For this review, use the dimensioned drawing (mm, ordinates from the lowest corner) and the shaded views. A direction names the side the tool comes from. Round coordinates to 2 decimals unless told otherwise and drop trailing zeros. Write each loop counter-clockwise with the first axis right and the second up, starting at its lowest first coordinate (ties: lowest second). Pieces come first, ordered by that corner, then holes. Notation, with made-up numbers: (84.5, -11.5) -> (130.5, -11.5) arc R31 ccw to (130.5, 27.5) -> close; hole circle Ø6 at (33.5, 46). An arc over 180 degrees is marked (long way). Write each question's results on one line, items separated by ' | '. Start each with the question number.
Item 1: Clearance check with flat-ended pins moving along their axes: pin 1 (15 mm diameter, centred on x = 19, z = 40.5, fed in from +Y); pin 2 (12 mm diameter, centred on x = 8.5, y = 15.5, fed in from -Z); pin 3 (10 mm diameter, centred on y = 27.5, z = 117.5, fed in from -X); pin 4 (4 mm diameter, centred on x = 29, y = 43, fed in from -Z). State where each tip first meets the part, or that it passes through.
Item 2: To check wall thickness, follow line 1 along Y through (x, z) = (33.9, 60); line 2 along Y through (x, z) = (19, 18); line 3 along X through (y, z) = (31.5, 63.5). State the ranges of each line that lie inside material, in increasing order.
Item 3: Add section C-C (z = 38.5). State the section outline as (x, y) points.
Item 4: Add section D-D (x = 19). State the section outline as (y, z) points.
Item 5: Tool access review of the marked faces 1 and 2: name each direction out of +Z, -Z, +X, -X, +Y, -Y from which nothing blocks a thin tool from reaching the whole face with its end or side.
Item 6: Add section B-B (y = 40). State the section outline as (x, z) points.
Item 7: Add section A-A (z = 61.5). State the section outline as (x, y) points, plus the area to 3 significant figures.
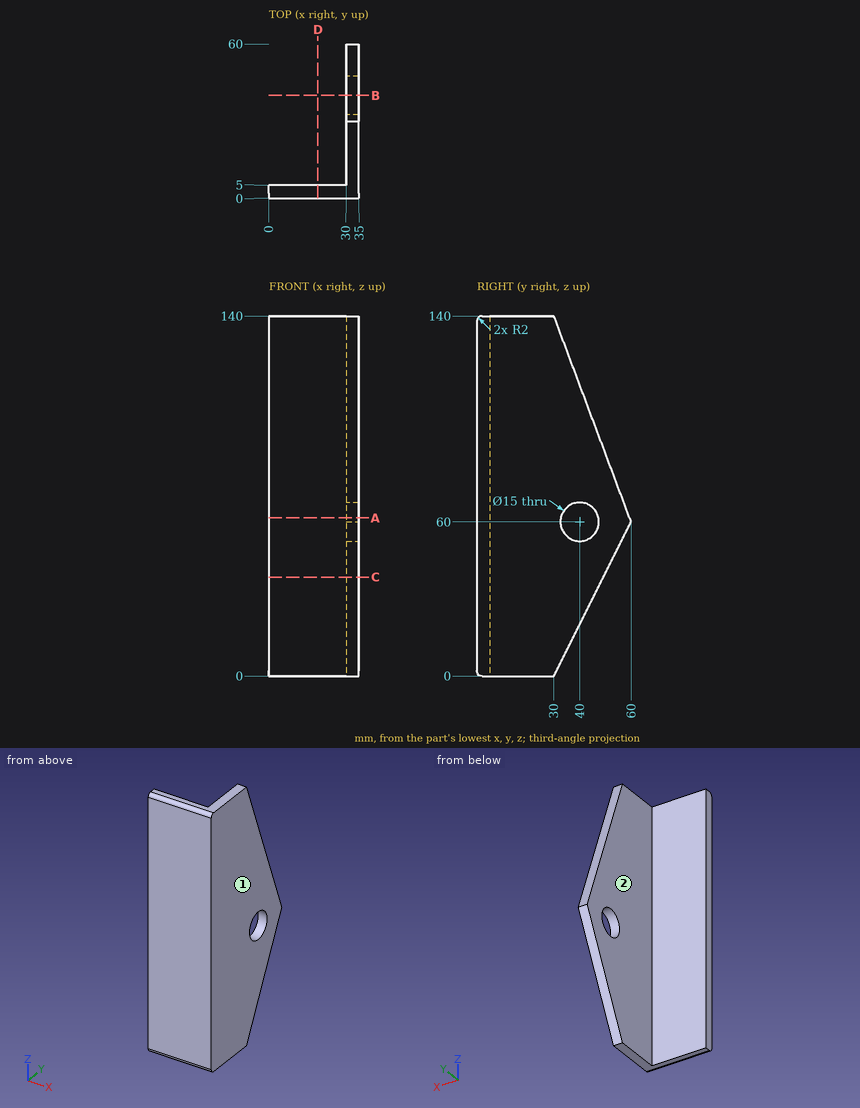
Responses:
1) pin 1: stops at y = 5 | pin 2: passes through | pin 3: stops at x = 30 | pin 4: stops at z = 22.54
2) line 1: y = 0 to 32.5, 47.5 to 60 | line 2: y = 0 to 5 | line 3: x = 30 to 35
3) outline: (0, 0) -> (35, 0) -> (35, 49.25) -> (30, 49.25) -> (30, 5) -> (0, 5) -> close
4) outline: (0, 2) arc R2 ccw to (2, 0) -> (5, 0) -> (5, 140) -> (2, 140) arc R2 ccw to (0, 138) -> close
5) face 1: +Z, -Z, +X, +Y, -Y | face 2: +Z, -Z, -X, +Y
6) outline: (30, 20) -> (35, 20) -> (35, 52.5) -> (30, 52.5) -> close; (30, 67.5) -> (35, 67.5) -> (35, 113.33) -> (30, 113.33) -> close
7) outline: (0, 0) -> (35, 0) -> (35, 32.65) -> (30, 32.65) -> (30, 5) -> (0, 5) -> close; (30, 47.35) -> (35, 47.35) -> (35, 59.44) -> (30, 59.44) -> close | area: 374 mm^2
